Input: dimensioned drawing with shaded views. Units: mm. Origin: part minimum x, y, z. A direction names the side the tool comes from. Coordinates: 2 decimals unless noted, no trailing zeros. Loops run counter-clockwise (first coordinate to the right, second up) from the corner with the lowest first, then second, coordinate; pieces in that order, holes last.
Item 1: Ray query, line 1 along Z through (x, y) = (7, 6); line 2 along X through (y, z) = (15.5, 80); line 3 along Z through (x, y) = (12.5, 29). Return the intervals inside material, ascending.
Item 2: Reachability of the marked faces 1 and 2 from +Z, -Z, +X, -X, +Y, -Y: full face, straight path, thin tool, end or side. Return the list, or none.
Item 3: Section D-D on z = 20. Return loops of the section in (x, y).
Item 4: Section C-C on z = 108. Return loops of the section in (x, y).
Item 5: Contact query for flat-ended pins moving along their axis: P1, Ø12, axis at x = 7.5, z = 93.5, coming from the +Y side; P2, Ø2, axis at x = 9, z = 95, coming from the +Y side; P3, Ø2, axis at y = 19.5, z = 28, coming from the -X side. Output: stop coordinate, or through.
Item 6: Section A-A on x = 15.31. Return loops of the section in (y, z), and give its area (3 significant figures).
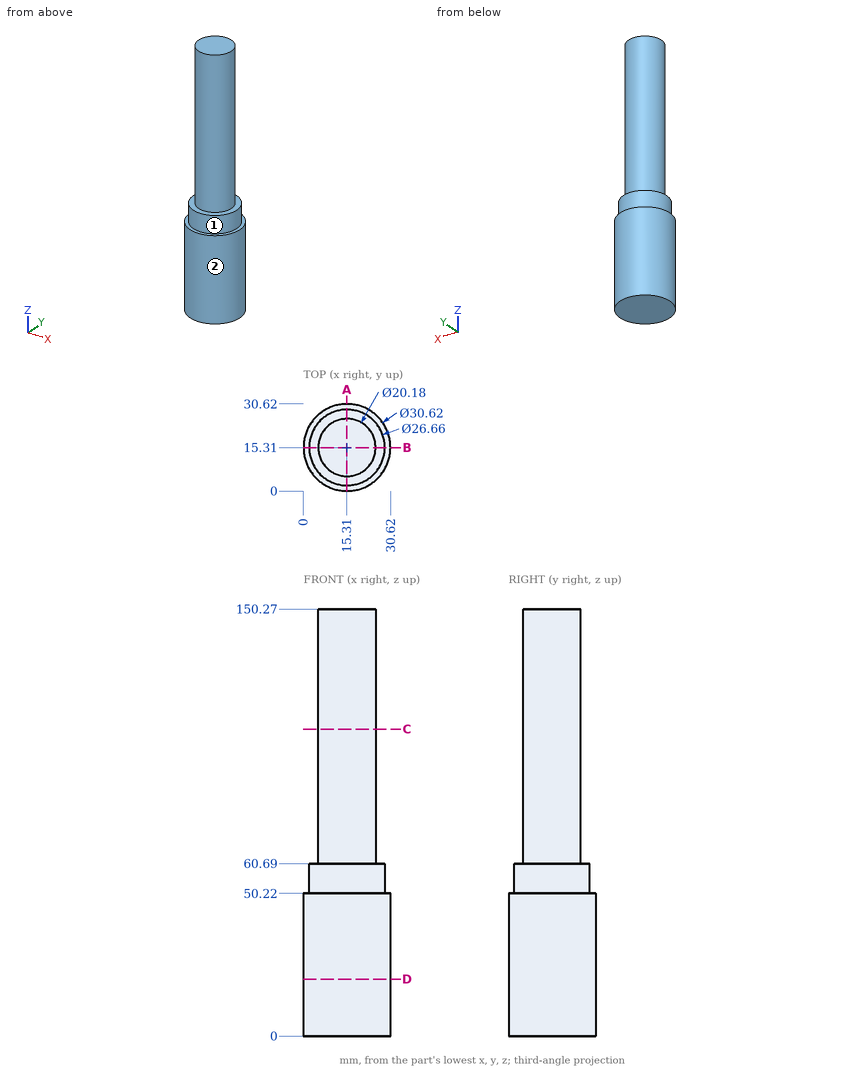
Results found:
1. line 1: z = 0 to 60.69
1. line 2: x = 5.22 to 25.4
1. line 3: z = 0 to 50.22
2. face 1: +Z
2. face 2: +Z, -Z
3. outline: circle Ø30.62 at (15.31, 15.31)
4. outline: circle Ø20.18 at (15.31, 15.31)
5. P1: stops at y = 25.24
5. P2: stops at y = 23.89
5. P3: stops at x = 0.34
6. outline: (0, 0) - (30.62, 0) - (30.62, 50.22) - (28.64, 50.22) - (28.64, 60.69) - (25.4, 60.69) - (25.4, 150.27) - (5.22, 150.27) - (5.22, 60.69) - (1.98, 60.69) - (1.98, 50.22) - (0, 50.22) - close
6. area: 3,620 mm2
